For this review, take the finished solid that the model builds, in its own axes (mm). Round coordinates to 2 decimals unless told otherwise and drop trailing zeros. Write each loop counter-clockwise with the first axis right and the second up, starting at its lowest first coordinate (ties: lowest second). Pieces come first, ordered by that corner, then holes. Notation, with made-up numbers: (-24.5, -21) -> (10.5, -21) arc R13 cw to (10.5, -8) -> close; hole circle Ø10 at (40.25, 51.25). An arc over 180 degrees is marked (long way). Write each question's results on one line, items separated by ' | '. Start each with the question number.
Item 1: Add section D-D (x = -38.5). State the section outline as (y, z) points.
Item 2: Clearance check with flat-ended pins moving along their axes: pin 1 (5 mm diameter, centred on x = -129, y = -3, fed in from +Z); pin 2 (3 mm diameter, centred on x = -38.5, y = -7.5, fed in from +Z); pin 3 (4 mm diameter, centred on x = 0, z = 0, fed in from -Y); pin 4 (5 mm diameter, centred on x = -122, y = -5, fed in from -Z). State where each tip first meets the part, or that it passes through.
Item 3: To check wall thickness, follow line 1 along Z through (x, y) = (0, -3.5); line 2 along Z through (x, y) = (-118, -9.5); line 3 along X through (y, z) = (-4.5, -70). State the ranges of each line that lie inside material, in increasing order.
Item 4: Add section C-C (y = -2.5). State the section outline as (x, z) points.
Item 5: Add section A-A (x = -159). State the section outline as (y, z) points.
Item 6: Add section B-B (z = 0). State the section outline as (x, y) points.
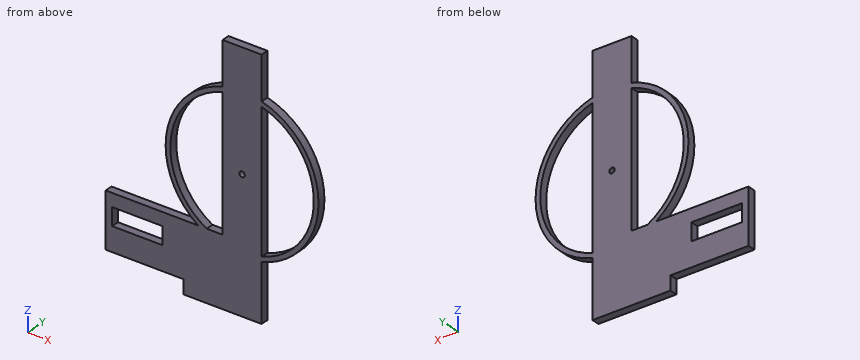
from build123d import *

# Parameters (mm, degrees)
F0_W      = 150
F0_H      = 70
F1_DEPTH  = 10
F2_R      = 98
F2_R_2    = 92
F3_DEPTH  = 10
F4_W      = 100
F4_H      = 10
F5_DEPTH  = 18
F6_R      = 3.5
F7_DEPTH  = 25
F8_R      = 3.5
F9_DEPTH  = 25
F10_W     = 65
F10_H     = 22.5
F11_DEPTH = 25


with BuildPart() as f1:
    # F0 (on Front) → F1 (new body)
    with BuildSketch(Plane.XZ):
        Polygon((25, 150), (-25, 150), (-25, -80), (-25, -150), (25, -150), align=None)
        with Locations((-100, -115)):
            Rectangle(F0_W, F0_H)
    extrude(amount=F1_DEPTH)

    # F2 (on face) → F3 (join)
    with BuildSketch(Plane.XZ.offset(10)):
        Circle(F2_R)
        Circle(F2_R_2, mode=Mode.SUBTRACT)
    extrude(amount=-F3_DEPTH)

    # F4 (on face) → F5 (join)
    with BuildSketch(Plane(origin=(0, 0, -150), x_dir=(1, 0, 0), z_dir=(0, 0, -1))):
        with Locations((-25, 5)):
            Rectangle(F4_W, F4_H)
    extrude(amount=F5_DEPTH)

    # F6 (on face) → F7 (cut)
    with BuildSketch(Plane.XZ.offset(10)):
        Circle(F6_R)
    extrude(amount=-F7_DEPTH, mode=Mode.SUBTRACT)

    # F8 (on face) → F9 (cut)
    with BuildSketch(Plane.XZ.offset(10)):
        with Locations((-113, -108)):
            Circle(F8_R)
    extrude(amount=-F9_DEPTH, mode=Mode.SUBTRACT)

    # F10 (on face) → F11 (cut)
    with BuildSketch(Plane.XZ.offset(10)):
        with Locations((-134.25, -108)):
            Rectangle(F10_W, F10_H)
    extrude(amount=-F11_DEPTH, mode=Mode.SUBTRACT)


solid = f1.part
Responses:
1) outline: (-10, -168) -> (0, -168) -> (0, -80) -> (-10, -80) -> close; (-10, 83.56) -> (0, 83.56) -> (0, 90.12) -> (-10, 90.12) -> close
2) pin 1: stops at z = -80 | pin 2: stops at z = 90.75 | pin 3: passes through | pin 4: stops at z = -150
3) line 1: z = -168 to -3.5, 3.5 to 150 | line 2: z = -150 to -119.25, -96.75 to -80 | line 3: x = -68.59 to -59.7, -25 to 25, 59.7 to 68.59
4) outline: (-175, -150) -> (-75, -150) -> (-75, -168) -> (25, -168) -> (25, -94.76) arc R98 ccw to (25, 94.76) -> (25, 150) -> (-25, 150) -> (-25, 94.76) arc R98 ccw to (-56.6, -80) -> (-175, -80) -> close; hole (-166.75, -119.25) -> (-101.75, -119.25) -> (-101.75, -96.75) -> (-166.75, -96.75) -> close; hole (-45.43, -80) -> (-25, -80) -> (-25, 88.54) arc R92 ccw to start; hole circle Ø7 at (0, 0); hole (25, -88.54) arc R92 ccw to (25, 88.54) -> close
5) outline: (-10, -150) -> (0, -150) -> (0, -119.25) -> (-10, -119.25) -> close; (-10, -96.75) -> (0, -96.75) -> (0, -80) -> (-10, -80) -> close
6) outline: (-98, -10) -> (-92, -10) -> (-92, 0) -> (-98, 0) -> close; (-25, -10) -> (-3.5, -10) -> (-3.5, 0) -> (-25, 0) -> close; (3.5, -10) -> (25, -10) -> (25, 0) -> (3.5, 0) -> close; (92, -10) -> (98, -10) -> (98, 0) -> (92, 0) -> close
